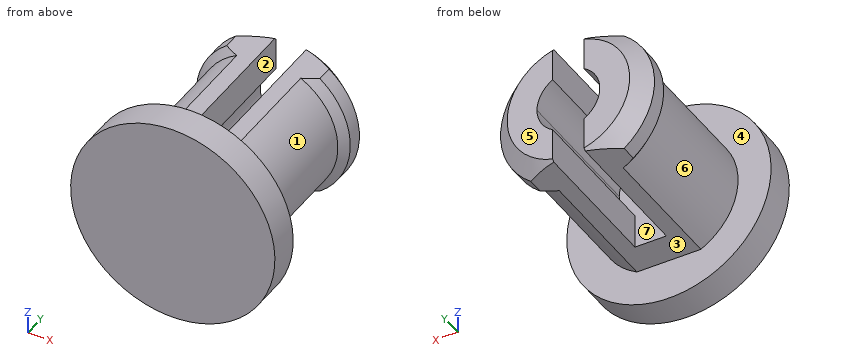
from build123d import *

# Parameters (mm, degrees)
ESBO_O1_R                = 6.5
RESSALTO_EXTRUS_O1_DEPTH = 2
ESBO_O2_R                = 4.4
RESSALTO_EXTRUS_O2_DEPTH = 8
ESBO_O3_R                = 4.9
RESSALTO_EXTRUS_O3_DEPTH = 3
CORTE_EXTRUS_O1_REACH    = 17.922
CORTE_EXTRUS_O2_DEPTH    = 9
CHANFRO1_SIZE            = 1


with BuildPart() as part:
    # Esboço1 → Ressalto-extrusão1 (new body)
    with BuildSketch(Plane(origin=(0, 0, 0), x_dir=(1, 0, 0), z_dir=(0, 1, 0))):
        with Locations(Location((0, 0, 0), (0, 0, 270))):
            Circle(ESBO_O1_R)
    extrude(amount=-RESSALTO_EXTRUS_O1_DEPTH)

    # Esboço2 → Ressalto-extrusão2 (add)
    with BuildSketch(Plane(origin=(0, 0, 0), x_dir=(1, 0, 0), z_dir=(0, 1, 0))):
        with Locations(Location((0, 0, 0), (0, 0, 270))):
            Circle(ESBO_O2_R)
    extrude(amount=RESSALTO_EXTRUS_O2_DEPTH)

    # Esboço3 → Ressalto-extrusão3 (add)
    with BuildSketch(Plane(origin=(0, 8, 0), x_dir=(1, 0, 0), z_dir=(0, 1, 0))):
        with Locations(Location((0, 0, 0), (0, 0, 270))):
            Circle(ESBO_O3_R)
    extrude(amount=RESSALTO_EXTRUS_O3_DEPTH)

    # Corte-extrusão1: up to this face of the body (flat: up to its plane)
    corte_extrus_o1_end = Plane(part.part.faces().sort_by_distance((0, 0, -6.316152237))[0])
    # Esboço4 → Corte-extrusão1 (cut, up to the picked face)
    with BuildSketch(Plane(origin=(0, 11, 0), x_dir=(1, 0, 0), z_dir=(0, 1, 0)), mode=Mode.PRIVATE) as corte_extrus_o1_sk1:
        with BuildLine():
            Line((2.966479395, -3.9), (-2.966479395, -3.9))
            ThreePointArc((-2.966479395, -3.9), (0, -4.9), (2.966479395, -3.9))
        make_face()
    corte_extrus_o1_tool1 = split(extrude(corte_extrus_o1_sk1.sketch, amount=-CORTE_EXTRUS_O1_REACH, mode=Mode.PRIVATE), bisect_by=corte_extrus_o1_end, keep=Keep.BOTH, mode=Mode.PRIVATE)
    # Esboço4 → Corte-extrusão1 (cut, up to the picked face)
    with BuildSketch(Plane(origin=(0, 11, 0), x_dir=(1, 0, 0), z_dir=(0, 1, 0)), mode=Mode.PRIVATE) as corte_extrus_o1_sk2:
        with BuildLine():
            ThreePointArc((2.966479395, 3.9), (0, 4.9), (-2.966479395, 3.9))
            Line((-2.966479395, 3.9), (2.966479395, 3.9))
        make_face()
    corte_extrus_o1_tool2 = split(extrude(corte_extrus_o1_sk2.sketch, amount=-CORTE_EXTRUS_O1_REACH, mode=Mode.PRIVATE), bisect_by=corte_extrus_o1_end, keep=Keep.BOTH, mode=Mode.PRIVATE)
    add(corte_extrus_o1_tool1.solids().sort_by(Axis((0, 11, 4.303719), (0, -1, 0)))[0], mode=Mode.SUBTRACT)
    add(corte_extrus_o1_tool2.solids().sort_by(Axis((0, 11, -4.303719), (0, -1, 0)))[0], mode=Mode.SUBTRACT)

    # Esboço5 → Corte-extrusão2 (cut)
    with BuildSketch(Plane(origin=(0, 11, 0), x_dir=(1, 0, 0), z_dir=(0, 1, 0))):
        with BuildLine():
            Line((0, 2), (0, 3.9))
            Line((0, 3.9), (-1, 3.9))
            Line((-1, 3.9), (-1, 1.732050808))
            ThreePointArc((-1, 1.732050808), (-0.51763809, 1.931851653), (0, 2))
        make_face()
        with BuildLine():
            Line((1, 3.9), (0, 3.9))
            Line((0, 3.9), (0, 2))
            ThreePointArc((0, 2), (0.51763809, 1.931851653), (1, 1.732050808))
            Line((1, 1.732050808), (1, 3.9))
        make_face()
        with BuildLine():
            Line((0, -3.9), (0, -2))
            ThreePointArc((0, -2), (-0.51763809, -1.931851653), (-1, -1.732050808))
            Line((-1, -1.732050808), (-1, -3.9))
            Line((-1, -3.9), (0, -3.9))
        make_face()
        with BuildLine():
            ThreePointArc((1, -1.732050808), (0.51763809, -1.931851653), (0, -2))
            Line((0, -2), (0, -3.9))
            Line((0, -3.9), (1, -3.9))
            Line((1, -3.9), (1, -1.732050808))
        make_face()
        with BuildLine():
            Line((0, -2), (0, 2))
            ThreePointArc((0, 2), (-0.51763809, 1.931851653), (-1, 1.732050808))
            Line((-1, 1.732050808), (-1, -1.732050808))
            ThreePointArc((-1, -1.732050808), (-0.51763809, -1.931851653), (0, -2))
        make_face()
        with BuildLine():
            ThreePointArc((1, 1.732050808), (0.51763809, 1.931851653), (0, 2))
            Line((0, 2), (0, -2))
            ThreePointArc((0, -2), (0.51763809, -1.931851653), (1, -1.732050808))
            Line((1, -1.732050808), (1, 1.732050808))
        make_face()
        with BuildLine():
            Line((-1, -1.732050808), (-1, 1.732050808))
            ThreePointArc((-1, 1.732050808), (-2, 0), (-1, -1.732050808))
        make_face()
        with BuildLine():
            ThreePointArc((2, 0), (1.732050808, 1), (1, 1.732050808))
            Line((1, 1.732050808), (1, -1.732050808))
            ThreePointArc((1, -1.732050808), (1.732050808, -1), (2, 0))
        make_face()
    extrude(amount=-CORTE_EXTRUS_O2_DEPTH, mode=Mode.SUBTRACT)

    # Chanfro1
    # the kernel refuses this chamfer: 1 mm, written as the material it takes off along each edge
    with BuildSketch(Plane(origin=(0, 8, 0), x_dir=(0.12482395655997021, 0, 0.9921789051722048), z_dir=(-0.9921789051722048, 0, 0.12482395655997021))) as chanfro1_piece_1_section:
        Polygon((4.9, CHANFRO1_SIZE), (4.9 - CHANFRO1_SIZE, 0), (4.9, 0), align=None)
    chanfro1_piece_1 = revolve(axis=Axis((0, 8, 0), (0, 1, 0)), revolution_arc=165.658820776, mode=Mode.PRIVATE)
    chanfro1_piece_1 = chanfro1_piece_1 - Plane(origin=(0, 8.751624074, 0), x_dir=(0, 0, 1), z_dir=(0, -1, 0)) * Cylinder(4.4, 20, mode=Mode.PRIVATE)
    add(chanfro1_piece_1, mode=Mode.SUBTRACT)
    with BuildSketch(Plane(origin=(0, 8, 0), x_dir=(-0.12482395656001569, 0, -0.9921789051721989), z_dir=(0.9921789051721989, 0, -0.12482395656001569))) as chanfro1_piece_2_section:
        Polygon((4.9 - CHANFRO1_SIZE, 0), (4.9, CHANFRO1_SIZE), (4.9, 0), align=None)
    chanfro1_piece_2 = revolve(axis=Axis((0, 8, 0), (0, 1, 0)), revolution_arc=165.658820776, mode=Mode.PRIVATE)
    chanfro1_piece_2 = chanfro1_piece_2 - Plane(origin=(0, 8.751624074, 0), x_dir=(0, 0, 1), z_dir=(0, -1, 0)) * Cylinder(4.4, 20, mode=Mode.PRIVATE)
    add(chanfro1_piece_2, mode=Mode.SUBTRACT)
    with BuildSketch(Plane(origin=(0, 11, 0), x_dir=(-0.124823956560002, 0, -0.9921789051722005), z_dir=(0.9921789051722005, 0, -0.124823956560002))) as chanfro1_piece_3:
        Polygon((4.9 - CHANFRO1_SIZE, 0), (4.9, -CHANFRO1_SIZE), (4.9, 0), align=None)
    revolve(axis=Axis((0, 11, 0), (0, 1, 0)), revolution_arc=165.658820776, mode=Mode.SUBTRACT)
    with BuildSketch(Plane(origin=(0, 11, 0), x_dir=(0.12482395656000247, 0, 0.9921789051722005), z_dir=(-0.9921789051722005, 0, 0.12482395656000247))) as chanfro1_piece_4:
        Polygon((4.9, -CHANFRO1_SIZE), (4.9 - CHANFRO1_SIZE, 0), (4.9, 0), align=None)
    revolve(axis=Axis((0, 11, 0), (0, 1, 0)), revolution_arc=165.658820776, mode=Mode.SUBTRACT)


solid = part.part
Geometry: final body of the model. Coordinates: model frame, mm. Face numbers are marked on the shaded views. A direction names the side the tool comes from. Round coordinates to 2 decimals unless told otherwise and drop trailing zeros. Write each loop counter-clockwise with the first axis right and the second up, starting at its lowest first coordinate (ties: lowest second). Pieces come first, ordered by that corner, then holes. Notation, with made-up numbers: M -14,-11 L 23,-11 A29 cw 23,18 Z; hole C 39.25,-8 d10. An arc over 180 degrees is marked long. Write item = value, one per line.
Item 1: Section query B-B on x = 0. Return loops of the section in (y, z).
Findings:
outline = M -2,-6.5 L 0,-6.5 L 0,-3.9 L 2,-3.9 L 2,3.9 L 0,3.9 L 0,6.5 L -2,6.5 Z
Item 2: Section query C-C on y = -1. Return loops of the section in (x, z), then the cut area to 3 significant figures.
Findings:
outline = C 0,0 d13
area = 133 mm^2
Item 3: Material intervals for line 1 along X through (y, z) = (8, -3.25); line 2 along Y through (x, z) = (-2, -4); line 3 along X through (y, z) = (7.5, -2.75), sorted ascending. Write a range as [from, to].
Findings:
line_1 = [-2.97, -1], [1, 2.97]
line_2 = [-2, 0]
line_3 = [-3.43, -1], [1, 3.43]
Item 4: Section query D-D on z = -5. Return loops of the section in (x, y).
Findings:
outline = M -4.15,-2 L 4.15,-2 L 4.15,0 L -4.15,0 Z
Item 5: Pin query (flat end, axial travel): P1, Ø0.7, axis at y = 5.5, z = -2.5, coming from the -X side; P2, Ø3, axis at x = -1.5, y = 6.5, coming from the +Z side; P3, Ø1.1, axis at y = 7.5, z = -2.5, coming from the +X side. Return the tip coordinate at first contact, or that it passes through.
Findings:
P1 = -3.84
P2 = 3.9
P3 = 3.94
Item 6: Section query A-A on y = 9.25. Return loops of the section in (x, z).
Findings:
outline = M -2.97,-3.9 L -1,-3.9 L -1,-1.73 A2 cw -1,1.73 L -1,3.9 L -2.97,3.9 A4.9 ccw Z; M 1,-3.9 L 2.97,-3.9 A4.9 ccw 2.97,3.9 L 1,3.9 L 1,1.73 A2 cw 1,-1.73 Z
Item 7: Access query for the marked faces 1, 2, 3 and 4. Directions: +Z, -Z, +X, -X, +Y, -Y. A direction counts if a zero-diameter tool reaches every point of the face in a straight line with its end or side. Return the directions, or none.
Findings:
face_1 = +X
face_2 = +Z, -Z, +Y
face_3 = -Z, +X, -X, +Y
face_4 = none
Item 8: Pull-direction query (Z, two-part tool) for the marked faces 5, 6 and 7; classes: pulls with the +Z half, pulls with the -Z half, needs draft (parallel to the pull), parting line crosses it, or undercut.
Findings:
face_5 = needs draft
face_6 = parting line crosses it
face_7 = undercut
